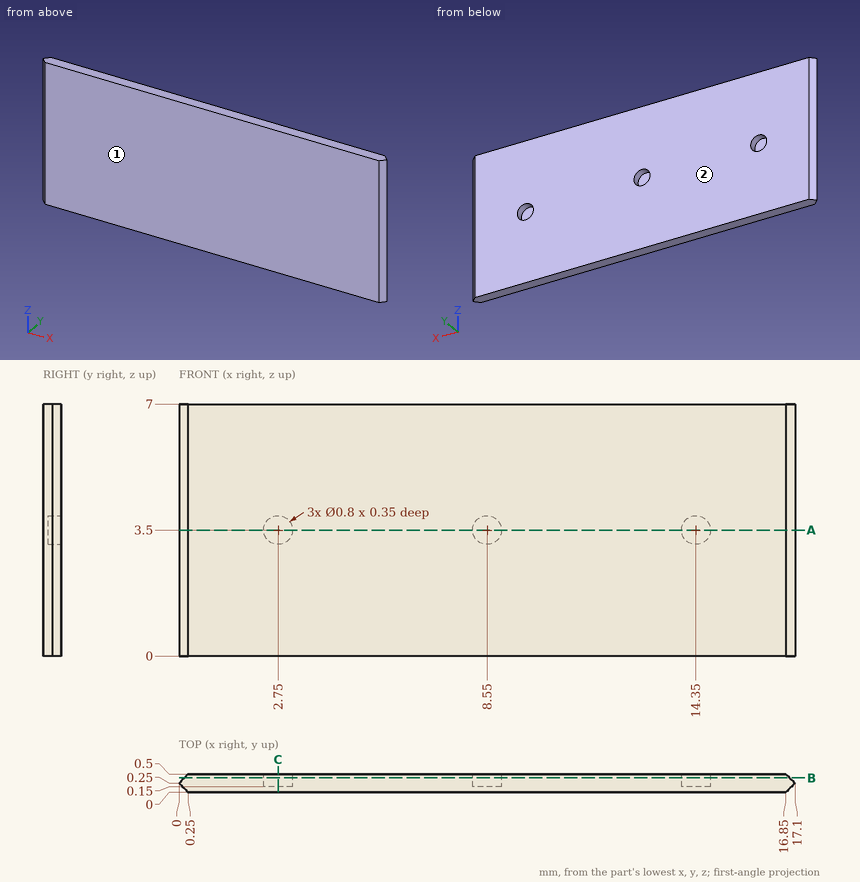
Drawing for the job (mm, zero at the part's lowest x, y, z). Round coordinates to 2 decimals unless told otherwise and drop trailing zeros. Loops run counter-clockwise (first coordinate to the right, second up) from the corner with the lowest first, then second, coordinate; pieces in that order, holes last. Notation, with made-up numbers: (25.25, -8.5) -> (71.25, -8.5) arc R23 cw to (71.25, 3.5) -> close; hole circle Ø10 at (-32, 3). An arc over 180 degrees is marked (long way). Answer in a Markdown table with one row per item.
Item 1: Drill centre lines: L1, parallel to Z at x = 2.75, y = 0.35; L2, parallel to X at y = 0.35, z = 3.5; L3, parallel to X at y = 0.4, z = 3.5. Where is each one in solid material? Low to high. Write a range as [from, to].
Answers below:
| item | result |
|---|---|
| L1 | z = [0, 3.1], [3.9, 7] |
| L2 | x = [0.1, 2.35], [3.15, 8.15], [8.95, 13.95], [14.75, 17] |
| L3 | x = [0.15, 2.35], [3.15, 8.15], [8.95, 13.95], [14.75, 16.95] |
Item 2: Saw through at A-A (z = 3.5). Write the cut outline in (x, y), and give its area (4 significant figures).
Answers below:
| item | result |
|---|---|
| outline | (0, 0.25) -> (0.25, 0) -> (16.85, 0) -> (17.1, 0.25) -> (16.85, 0.5) -> (14.75, 0.5) -> (14.75, 0.15) -> (13.95, 0.15) -> (13.95, 0.5) -> (8.95, 0.5) -> (8.95, 0.15) -> (8.15, 0.15) -> (8.15, 0.5) -> (3.15, 0.5) -> (3.15, 0.15) -> (2.35, 0.15) -> (2.35, 0.5) -> (0.25, 0.5) -> close |
| area | 7.585 mm² |
Item 3: Saw through at B-B (y = 0.4). Write the cut outline in (x, z), and give its area (3 significant figures).
Answers below:
| item | result |
|---|---|
| outline | (0.15, 0) -> (16.95, 0) -> (16.95, 7) -> (0.15, 7) -> close; hole circle Ø0.8 at (2.75, 3.5); hole circle Ø0.8 at (8.55, 3.5); hole circle Ø0.8 at (14.35, 3.5) |
| area | 116 mm² |
Item 4: Mould opens along Y. For the marked faces 1 and 2 say: +Y half, -Y half, draft (parallel to the pull), parting line (faces both ways), or undercut.
Answers below:
| item | result |
|---|---|
| face 1 | -Y half |
| face 2 | +Y half |
Item 5: Saw through at C-C (x = 2.75). Write the cut outline in (y, z).
Answers below:
| item | result |
|---|---|
| outline | (0, 0) -> (0.5, 0) -> (0.5, 3.1) -> (0.15, 3.1) -> (0.15, 3.9) -> (0.5, 3.9) -> (0.5, 7) -> (0, 7) -> close |
